For this review, take the finished solid that the model builds, in its own axes (mm). Face numbers are marked on the shaded views. A direction names the side the tool comes from. Coordinates: 2 decimals unless noted, no trailing zeros. Write each loop counter-clockwise with the first axis right and the second up, starting at its lowest first coordinate (ties: lowest second). Pieces come first, ordered by that corner, then holes. Notation, with made-up numbers: M 38.25,65 L 48.25,65 A33 cw 48.25,104 Z; hole C 74.25,-9 d6. An arc over 180 degrees is marked long. One line per question, with ' | ' between items.
from build123d import *

# Parameters (mm, degrees)
REVOLVE1_ANGLE = 270


with BuildPart() as part:
    # Sketch1 → Revolve1 (revolve)
    with BuildSketch(Plane.XY):
        Polygon((-40, 192.728692059), (-80, 192.728692059), (-80, 142.728692059), (-125, 142.728692059), (-125, 92.728692059), (-205, 92.728692059), (-205, -47.271307941), (-125, -47.271307941), (-125, -107.271307941), (-60, -107.271307941), (-60, -7.271307941), (-155, -7.271307941), (-155, 57.728692059), (-75, 57.728692059), (-75, 107.728692059), (-40, 107.728692059), align=None)
    revolve(axis=Axis((0, -107.271307941, 0), (0, 1, 0)), revolution_arc=REVOLVE1_ANGLE)


solid = part.part
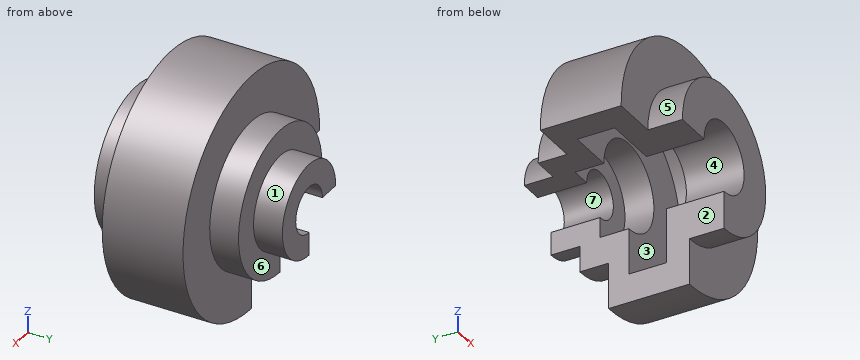
1. Clearance check with flat-ended pins moving along their axes: P1, Ø6, axis at x = 24, z = -81.5, coming from the +Y side; P2, Ø1.5, axis at y = 91, z = -135.5, coming from the -X side; P3, Ø2, axis at y = 92.5, z = 147.5, coming from the -X side. State where each tip first meets the part, or that it passes through.
Computed values:
P1: stops at y = 142.73 | P2: stops at x = 0 | P3: stops at x = -143.4
2. Draft analysis for pull direction Z (two halves, no side actions). For the marked faces 5, 6 and 7, state which applies: pulls with the +Z half, pulls with the -Z half, needs draft (parallel to the pull), parting line crosses it, or undercut.
Computed values:
face 5: parting line crosses it | face 6: needs draft | face 7: undercut
3. Take a section at B-B on x = 92. State the section outline as (y, z) points.
Computed values:
outline: M -107.27,-84.62 L -47.27,-84.62 L -47.27,-183.2 L 92.73,-183.2 L 92.73,-84.62 L 142.73,-84.62 L 142.73,84.62 L 92.73,84.62 L 92.73,183.2 L -47.27,183.2 L -47.27,84.62 L -107.27,84.62 Z; hole M -7.27,-124.74 L 57.73,-124.74 L 57.73,124.74 L -7.27,124.74 Z
4. Machinability: for the marked faces 1, 2, 3 and 4, which of the approach directions +Z, -Z, +X, -X, +Y, -Y give a long, thin tool a straight path to every point of the face, cutting with its end or side? Answer none if there is none.
Computed values:
face 1: +Y | face 2: -Z, -X, +Y, -Y | face 3: none | face 4: -Y
5. Take a section at D-D on x = -143.5. State the section outline as (y, z) points.
Computed values:
outline: M -47.27,0 L -7.27,0 L -7.27,58.59 L 57.73,58.59 L 57.73,0 L 92.73,0 L 92.73,146.4 L -47.27,146.4 Z
6. For line 1 along Y through (x, z) = (96, -59); line 2 along Y through (x, z) = (66, 10.5); line 3 along Y through (x, z) = (126.5, -161), list the stretches that pass through material, from the lowest coordinate up.
Computed values:
line 1: y = -107.27 to -7.27, 57.73 to 142.73 | line 2: y = -107.27 to -7.27, 107.73 to 192.73 | line 3: y = -47.27 to 92.73
7. Take a section at C-C on z = 141. State the section outline as (x, y) points, plus the area to 3 significant figures.
Computed values:
outline: M -148.81,-47.27 L 148.81,-47.27 L 148.81,92.73 L -148.81,92.73 Z; hole M -64.37,-7.27 L 64.37,-7.27 L 64.37,57.73 L -64.37,57.73 Z | area: 33,300 mm2
